from build123d import *

# Parameters (mm, degrees)
SKETCH1_R               = 7.14375
BOSS_EXTRUDE1_DEPTH     = 14.2875
SKETCH2_R               = 3.175
CUT_EXTRUDE1_DEPTH      = 12.7
SKETCH3_W               = 14.2875
SKETCH3_H               = 7.62
CUT_EXTRUDE2_DEPTH      = 14.2875
CUT_EXTRUDE4_DEPTH      = 18.49854235
CUT_EXTRUDE4_DEPTH_BACK = 18.49854235
CUT_EXTRUDE5_DEPTH      = 18.49854252
CUT_EXTRUDE5_DEPTH_BACK = 18.49854252
SKETCH5_R               = 1.5875
SKETCH6_R               = 1.5875
CUT_EXTRUDE6_DEPTH      = 12.7


with BuildPart() as part:
    # Sketch1 → Boss-Extrude1 (new, symmetric)
    with BuildSketch(Plane(origin=(0, 0, 0), x_dir=(1, 0, 0), z_dir=(0, 1, 0))):
        with Locations(Location((0, 0, 0), (0, 0, 270))):
            Circle(SKETCH1_R)
    extrude(amount=BOSS_EXTRUDE1_DEPTH, both=True)

    # Sketch2 → Cut-Extrude1 (cut)
    with BuildSketch(Plane.XZ.offset(14.2875)):
        with Locations(Location((0, 0, 0), (0, 0, 270))):
            Circle(SKETCH2_R)
    extrude(amount=-CUT_EXTRUDE1_DEPTH, mode=Mode.SUBTRACT)

    # Sketch3 → Cut-Extrude2 (cut)
    with BuildSketch(Plane(origin=(0, 14.2875, 0), x_dir=(1, 0, 0), z_dir=(0, 1, 0))):
        Rectangle(SKETCH3_W, SKETCH3_H)
    extrude(amount=-CUT_EXTRUDE2_DEPTH, mode=Mode.SUBTRACT)

    # Sketch4 → Cut-Extrude4 (cut, two sides: drawn at the far end of the back side and taken through both)
    with BuildSketch(Plane.XY.offset(-CUT_EXTRUDE4_DEPTH_BACK)):
        with BuildLine():
            Line((-57.554902545, 0), (-7.14375, 0))
            Line((-7.14375, 0), (-5.87375, 0))
            Line((-5.87375, 0), (-5.062065416, 9.633990007))
            ThreePointArc((-5.062065416, 9.633990007), (0, 14.2875), (5.062065416, 9.633990007))
            Line((5.062065416, 9.633990007), (5.87375, 0))
            Line((5.87375, 0), (7.14375, 0))
            Line((7.14375, 0), (57.554902545, 0))
            Line((57.554902545, 0), (57.554902545, 100.82230509))
            Line((57.554902545, 100.82230509), (-57.554902545, 100.82230509))
            Line((-57.554902545, 100.82230509), (-57.554902545, 0))
        make_face()
    extrude(amount=CUT_EXTRUDE4_DEPTH + CUT_EXTRUDE4_DEPTH_BACK, mode=Mode.SUBTRACT)

    # Sketch5 → Cut-Extrude5 (cut, two sides: drawn at the far end of the back side and taken through both)
    with BuildSketch(Plane.XY.offset(-CUT_EXTRUDE5_DEPTH_BACK)):
        with Locations(Location((0, 11.1125, 0), (0, 0, 90))):
            Circle(SKETCH5_R)
    extrude(amount=CUT_EXTRUDE5_DEPTH + CUT_EXTRUDE5_DEPTH_BACK, mode=Mode.SUBTRACT)

    # Sketch6 → Cut-Extrude6 (cut, symmetric)
    with BuildSketch(Plane(origin=(0, 0, 0), x_dir=(0, 0, -1), z_dir=(1, 0, 0))):
        with Locations((0, -7.9375)):
            Circle(SKETCH6_R)
    extrude(amount=CUT_EXTRUDE6_DEPTH, both=True, mode=Mode.SUBTRACT)


solid = part.part
Model file for the job. Use its own axes, mm. A direction names the side the tool comes from. Round coordinates to 2 decimals unless told otherwise and drop trailing zeros. Order: outer loops, then holes, each group sorted by start corner. A loop starts at its lowest first (then second) coordinate and runs counter-clockwise, first axis right, second up. Notation, with made-up numbers: M -19.5,34 L 13.5,34 A21 cw 13.5,67 Z; hole C 74,-20.5 d9. An arc over 180 degrees is marked long. Write each question's results on one line, items separated by ' | '. Start each with the question number.
(1) Drop flat-ended pins along their axis: pin 1 (6 mm diameter, centred on y = -5.5, z = -4, fed in from +X); pin 2 (1.5 mm diameter, centred on x = -5, z = 0.5, fed in from +Y); pin 3 (3 mm diameter, centred on x = 0, y = 11.11, fed in from +Z); pin 4 (6 mm diameter, centred on x = 5, y = 0.5, fed in from -Z). Give the stop position or say it passes through.
(2) Probe probe 1 along Y at (x, z) = (0, 5.85) (1 decimal); probe 2 along Y at (x, z) = (-0.75, 3.5); probe 3 along Z at (x, y) = (1.5, 5). List the from-to ranges inside material, lowest first. Write a range as from..to.
(3) Saw through at A-A, the plane x = 0. Give the cut face in (y, z) (1 decimal).
(4) Which spindle directions (+Z, -Z, +X, -X, +Y, -Y) get a long thin tool onto all of the face, cutting with end or side? Do faces 1 (the face through (0, 6, -3.81)), 2 (the face through (-1.22, -8.03, -2.93)), 3 (the face through (-5.383, 5.82, -4.297)). Say none if no direction does.
(5) Saw through at B-B, the plane z = 0. State how many separate pieces and enclosed holes the cut face has, then the cut area to 3 significant figures.
(6) Saw through at C-C, the plane y = 5.5. Give the cut face in (x, z), then the cut area to 3 significant figures.
(7) Two-plate mould, pull along Z, no slides. Class faces 4 (the face through (0, -1.588, 0)), 5 (the face through (0.314, -2.974, -7.137)), 6 (the face through (-1.5, -14.288, 3.1)): pulls with the +Z half, pulls with the -Z half, needs draft (parallel to the pull), parting line crosses it, or undercut.
Established:
1) pin 1: stops at x = 7.07 | pin 2: stops at y = 0 | pin 3: passes through | pin 4: stops at z = -6.86
2) probe 1: y = -14.3..9.5, 12.7..14.3 | probe 2: y = -14.29..0 | probe 3: z = -6.98..-3.81, 3.81..6.98
3) outline: M -14.3,-7.1 L 9.5,-7.1 L 9.5,-3.8 L 0,-3.8 L 0,3.8 L 9.5,3.8 L 9.5,7.1 L -14.3,7.1 L -14.3,3.2 L -1.6,3.2 L -1.6,-3.2 L -14.3,-3.2 Z; M 12.7,-7.1 L 14.3,-7.1 L 14.3,-3.8 L 12.7,-3.8 Z; M 12.7,3.8 L 14.3,3.8 L 14.3,7.1 L 12.7,7.1 Z
4) face 1: +X, -X, +Y | face 2: -Y | face 3: +Z, -Z, -X, +Y
5) separate pieces: 3 | enclosed holes: 0 | area: 98.3 mm^2
6) outline: M -5.41,-4.66 A7.14 ccw 5.41,-4.66 L 5.41,-3.81 L -5.41,-3.81 Z; M -5.41,3.81 L 5.41,3.81 L 5.41,4.66 A7.14 ccw -5.41,4.66 Z | area: 55.7 mm^2
7) face 4: undercut | face 5: parting line crosses it | face 6: needs draft
